from build123d import *

# Parameters (mm, degrees)
SKETCH1_R           = 1.5
BOSS_EXTRUDE1_DEPTH = 3
BOSS_EXTRUDE2_START = 22.5
SKETCH2_W           = 3.5
SKETCH2_H           = 6
BOSS_EXTRUDE2_DEPTH = 29
SKETCH4_R           = 1.5
BOSS_EXTRUDE5_DEPTH = 1
CHAMFER2_SIZE       = 2
CHAMFER2_SIZE2      = 3.464101615
SKETCH3_W           = 24
SKETCH3_H           = 29
SKETCH3_R           = 11
BOSS_EXTRUDE4_DEPTH = 7
CHAMFER3_SIZE       = 2
SKETCH5_R           = 2
BOSS_EXTRUDE6_DEPTH = 14


# Read off the part's stored shape, not the designer's step: Mirror1
with BuildPart() as part:
    # Sketch1 → Boss-Extrude1 (new body)
    with BuildSketch(Plane(origin=(0, 0, 0), x_dir=(1, 0, 0), z_dir=(0, 1, 0))):
        Polygon((-6, 17), (-3, 20), (3, 20), (6, 17), (6, -17), (3, -20), (-3, -20), (-6, -17), align=None)
        with Locations(Location((0, 14, 0), (0, 0, 270))):
            Circle(SKETCH1_R, mode=Mode.SUBTRACT)
        with Locations(Location((0, -14, 0), (0, 0, 270))):
            Circle(SKETCH1_R, mode=Mode.SUBTRACT)
    extrude(amount=BOSS_EXTRUDE1_DEPTH)

    # Sketch2 → Boss-Extrude2 (add)
    with BuildSketch(Plane(origin=(0, 3, 0), x_dir=(1, 0, 0), z_dir=(0, 1, 0)).offset(BOSS_EXTRUDE2_START)):
        with Locations((-7.75, 9)):
            Rectangle(SKETCH2_W, SKETCH2_H)
        with Locations((-7.75, -9)):
            Rectangle(SKETCH2_W, SKETCH2_H)
    extrude(amount=-BOSS_EXTRUDE2_DEPTH)

    # Sketch4 → Boss-Extrude5 (add)
    with BuildSketch(Plane(origin=(0, 3, 0), x_dir=(1, 0, 0), z_dir=(0, 1, 0))):
        Polygon((-3, 20), (-6, 17), (-6, 12), (-6, 6), (-6, -6), (-6, -12), (-6, -17), (-3, -20), (3, -20), (6, -17), (6, 17), (3, 20), align=None)
        with Locations(Location((0, 14, 0), (0, 0, 270))):
            Circle(SKETCH4_R, mode=Mode.SUBTRACT)
        with Locations(Location((0, -14, 0), (0, 0, 270))):
            Circle(SKETCH4_R, mode=Mode.SUBTRACT)
    extrude(amount=BOSS_EXTRUDE5_DEPTH)

    # Chamfer2
    chamfer2_edges = [part.edges().sort_by_distance(p)[0] for p in [
        (-6, 0, -9),
        (-6, 0, 9),
    ]]
    chamfer2_side = [part.faces().sort_by_distance(p)[0] for p in [
        (0, 0, 0),
    ]]
    chamfer(chamfer2_edges, length=CHAMFER2_SIZE, length2=CHAMFER2_SIZE2, reference=chamfer2_side[0])

    # Sketch3 → Boss-Extrude4 (add)
    with BuildSketch(Plane.ZY.offset(9.5)):
        with Locations((0, 11)):
            Rectangle(SKETCH3_W, SKETCH3_H)
        with Locations(Location((0, 11, 0), (0, 0, 236.944268849))):
            Circle(SKETCH3_R, mode=Mode.SUBTRACT)
    extrude(amount=BOSS_EXTRUDE4_DEPTH)

    # Chamfer3
    chamfer3_edges = [part.edges().sort_by_distance(p)[0] for p in [
        (-11.25, 25.5, -12),
        (-11.25, -3.5, -12),
        (-11.25, -3.5, 12),
        (-11.25, 25.5, 12),
    ]]
    chamfer(chamfer3_edges, length=CHAMFER3_SIZE)

    # Mirror1: part across plane


with BuildPart() as part_1:
    add(part.part)
    add(part.part.mirror(Plane(origin=(0, 11, 0), x_dir=(0, 0, 1), z_dir=(0, -1, 0))))

    # Sketch5 → Boss-Extrude6 (add)
    # profile 1 of 2: a face of its own
    with BuildSketch(Plane(origin=(0, 4, 0), x_dir=(1, 0, 0), z_dir=(0, 1, 0))):
        Polygon((6, -6), (-6, -6), (-6, -17), (-3, -20), (3, -20), (6, -17), align=None)
        with Locations(Location((0, -14, 0), (0, 0, 90))):
            Circle(SKETCH5_R, mode=Mode.SUBTRACT)
    # profile 2 of 2: a face of its own
    with BuildSketch(Plane(origin=(0, 4, 0), x_dir=(1, 0, 0), z_dir=(0, 1, 0))):
        Polygon((-6, 17), (-6, 6), (6, 6), (6, 17), (3, 20), (-3, 20), align=None)
        with Locations(Location((0, 14, 0), (0, 0, 90))):
            Circle(SKETCH5_R, mode=Mode.SUBTRACT)
    extrude(amount=BOSS_EXTRUDE6_DEPTH)


solid = part_1.part
Part model, mm, in its own coordinate system. A direction names the side the tool comes from. Give positions to 0.01 mm unless a question says otherwise; leave off trailing zeros. Order: outer loops, then holes, each group sorted by start corner. A loop starts at its lowest first (then second) coordinate and runs counter-clockwise, first axis right, second up. Notation, with made-up numbers: (-5, 87.5) -> (35, 87.5) arc R25 cw to (35, 113.5) -> close; hole circle Ø10 at (-24.75, -3.5). An arc over 180 degrees is marked (long way). Use one line per item in the form item = value.
(1) Saw through at C-C (z = 0). Write the cut outline in (x, y).
Solution:
outline = (-16.5, -3.5) -> (-9.5, -3.5) -> (-9.5, 0) -> (-16.5, 0) -> close; (-16.5, 22) -> (-9.5, 22) -> (-9.5, 25.5) -> (-16.5, 25.5) -> close; (-6, 0) -> (6, 0) -> (6, 4) -> (-6, 4) -> close; (-6, 18) -> (6, 18) -> (6, 22) -> (-6, 22) -> close
(2) Flat gauge pins, fed straight in: P1, Ø4.5, axis at x = 0, z = 14, coming from the +Y side; P2, Ø6, axis at x = 1, z = -3.5, coming from the -Y side; P3, Ø2.5, axis at x = 0, z = 14, coming from the +Y side; P4, Ø9.5, axis at x = -0.5, z = 9.5, coming from the -Y side. Where does each tip first touch, or does it go through?
Solution:
P1 = 22
P2 = 0
P3 = through
P4 = -2.17
(3) Pull direction Z, two halves, no side cores. Call faces 1 (the face through (0, 11, -20)), 2 (the face through (-5, 11, 18)), 3 (the face through (0, 18, 0)): +Z half, -Z half, draft (parallel to the pull), parting line (faces both ways), or undercut.
Solution:
face_1 = -Z half
face_2 = +Z half
face_3 = undercut
(4) Saw through at B-B (y = 11). Write the cut outline in (x, z).
Solution:
outline = (-16.5, -12) -> (-6, -12) -> (-6, -17) -> (-3, -20) -> (3, -20) -> (6, -17) -> (6, -6) -> (-9.5, -6) -> (-9.5, -11) -> (-16.5, -11) -> close; (-16.5, 11) -> (-9.5, 11) -> (-9.5, 6) -> (6, 6) -> (6, 17) -> (3, 20) -> (-3, 20) -> (-6, 17) -> (-6, 12) -> (-16.5, 12) -> close; hole circle Ø4 at (0, -14); hole circle Ø4 at (0, 14)
(5) Saw through at A-A (x = 0). Count the separate pieces of the cut face and the enclosed holes in it, then the cut area to 3 significant figures.
Solution:
separate_pieces = 3
enclosed_holes = 1
area = 552 mm²
(6) Tool access for faces 4 (the face through (-6, 11, -15)), 5 (the face through (-9.5, 11, -8)), 6 (the face through (1.2, 10.9, -12.4)): list every direction of +Z, -Z, +X, -X, +Y, -Y with a clear straight run to the whole face (end or side of a thin tool).
Solution:
face_4 = -Z, -X, +Y, -Y
face_5 = -X
face_6 = none
(7) Drill centre lines: line 1 (Y direction, x = -14, z = 0); line 2 (Z direction, x = -3, y = 17); line 3 (Z direction, x = -8.5, y = 1.75). Where is each one in solid material? Low to high. Write a range as from..to.
Solution:
line_1 = -3.5..0, 22..25.5
line_2 = -20..-6, 6..20
line_3 = -12..-6, 6..12
(8) Saw through at D-D (x = -7.5). Write the cut outline in (y, z), then the cut area to 3 significant figures.
Solution:
outline = (-3.5, -10) -> (-1.5, -12) -> (23.5, -12) -> (25.5, -10) -> (25.5, -6) -> (-3.5, -6) -> close; (-3.5, 6) -> (25.5, 6) -> (25.5, 10) -> (23.5, 12) -> (-1.5, 12) -> (-3.5, 10) -> close
area = 340 mm²
